Read the model definition and answer for the solid it produces. Units are mm, in the model's axes. A direction names the side the tool comes from. Coordinates: 2 decimals unless noted, no trailing zeros. Write each loop counter-clockwise with the first axis right and the second up, starting at its lowest first coordinate (ties: lowest second). Pieces come first, ordered by that corner, then holes.
1) The part is cut by section D-D (y = -12.25). Determine the outline of the cut face in (x, z).
2) Which of the six approach directions +Z, -Z, +X, -X, +Y, -Y give full straight-line access (tool end or side, diameter ignored) to faces 5 (the face through (7.5, -8, 12)), 6 (the face through (5.5, -6, 12)), 7 (the face through (0, -14.5, 10))?
3) Find the intervals of material crossed by line 1 (X direction, y = -4.5, z = 17); line 2 (Z direction, x = 0, y = -13.4); line 3 (X direction, y = 5.5, z = 11.25), in increasing order.
4) Determine the mould class of faces 1 (the face through (-10.215, 12.199, 12.325)), 2 (the face through (-10, 0, 12)), 3 (the face through (-11.9, 13.93, 12.32)), 4 (the face through (10.199, 12.215, 12.325)) for opening direction X: +X half, -X half, draft (parallel to the pull), parting line (faces both ways), or undercut.
5) Each of these flat-tipped pins is pushed along its axis until it touches: pin 1 Ø6 at (y, z) = (-7, 13.5) entering from +X; pin 2 Ø5.5 at (x, z) = (-1, 12.5) entering from +Y; pin 3 Ø2.5 at (y, z) = (-8.5, 14) entering from -X. Where does it stop, or does it pass through?
6) The part is cut by section C-C (y = 6.5). Determine the outline of the cut face in (x, z), then the cut area to 3 significant figures.
7) The part is cut by section B-B (x = 0). Determine the outline of the cut face in (y, z), then the cut area to 3 significant figures.
from build123d import *

# Parameters (mm, degrees)
F1_DEPTH    = 25
F2_R        = 1.85
F3_DEPTH    = 16.3
F4_T1_DEPTH = 25
F7_R        = 4
F5_DEPTH    = 8.1194955856
F6_DEPTH    = 1.5


# Not quite as in the source:
# - a fillet or chamfer that OpenCascade refuses, or shapes differently, is made with other operations: its cross-section is extruded or revolved along the edge and cut away or added


with BuildPart() as f1:
    # F0 (on Top) → F1 (new body)
    with BuildSketch(Plane.XY):
        with BuildLine():
            Line((-7.5, -2), (-7.5, -14.5))
            Line((-7.5, -14.5), (7.5, -14.5))
            Line((7.5, -14.5), (7.5, -2))
            ThreePointArc((7.5, -2), (8.0857864376, -0.5857864376), (9.5, 0))
            Line((9.5, 0), (10.5, 0))
            ThreePointArc((10.5, 0), (11.9142135624, 0.5857864376), (12.5, 2))
            Line((12.5, 2), (12.5, 12.5))
            ThreePointArc((12.5, 12.5), (11.9142135624, 13.9142135624), (10.5, 14.5))
            Line((10.5, 14.5), (-10.5, 14.5))
            ThreePointArc((-10.5, 14.5), (-11.9142135624, 13.9142135624), (-12.5, 12.5))
            Line((-12.5, 12.5), (-12.5, 2))
            ThreePointArc((-12.5, 2), (-11.9142135624, 0.5857864376), (-10.5, 0))
            Line((-10.5, 0), (-9.5, 0))
            ThreePointArc((-9.5, 0), (-8.0857864376, -0.5857864376), (-7.5, -2))
        make_face()
        with BuildLine():
            Line((-10.5, 1.8729833462), (-10.5, 12.5))
            Line((-10.5, 12.5), (10.5, 12.5))
            Line((10.5, 12.5), (10.5, 1.8729833462))
            ThreePointArc((10.5, 1.8729833462), (7.0505102572, 1.1622776602), (5.5, -2))
            Line((5.5, -2), (5.5, -12.5))
            Line((5.5, -12.5), (-5.5, -12.5))
            Line((-5.5, -12.5), (-5.5, -2))
            ThreePointArc((-5.5, -2), (-7.0505102572, 1.1622776602), (-10.5, 1.8729833462))
        make_face(mode=Mode.SUBTRACT)
    extrude(amount=F1_DEPTH)

    # F2 (on face) → F3 (cut)
    with BuildSketch(Plane.XZ.offset(14.5)):
        with Locations((0, 12.5)):
            Circle(F2_R)
    extrude(amount=-F3_DEPTH, mode=Mode.SUBTRACT)

    # F4: fillet of radius 1 on 4 edges, made by hand

    # F4_s2 → F4_t1 (join)
    with BuildSketch(Plane.XY):
        with BuildLine():
            ThreePointArc((-10.5, 11.5), (-10.2071067812, 12.2071067812), (-9.5, 12.5))
            Line((-9.5, 12.5), (-10.5, 12.5))
            Line((-10.5, 12.5), (-10.5, 11.5))
        make_face()
        with BuildLine():
            ThreePointArc((9.5, 12.5), (10.2071067812, 12.2071067812), (10.5, 11.5))
            Line((10.5, 11.5), (10.5, 12.5))
            Line((10.5, 12.5), (9.5, 12.5))
        make_face()
        with BuildLine():
            ThreePointArc((9.5, 2), (10.2071067812, 2.2928932188), (10.5, 3))
            Line((10.5, 3), (10.5, 1.8729833462))
            ThreePointArc((10.5, 1.8729833462), (10.0040171699, 1.9681187851), (9.5, 2))
        make_face()
        with BuildLine():
            ThreePointArc((-9.5, 2), (-10.2071067812, 2.2928932188), (-10.5, 3))
            Line((-10.5, 3), (-10.5, 1.8729833462))
            ThreePointArc((-10.5, 1.8729833462), (-10.0040171699, 1.9681187851), (-9.5, 2))
        make_face()
    extrude(amount=F4_T1_DEPTH)

    # F7 (on face) → F5 (cut)
    with BuildSketch(Plane(origin=(0, 14.5, 0), x_dir=(-1, 0, 0), z_dir=(0, 1, 0))):
        with Locations((0, 12.5)):
            Circle(F7_R)
    extrude(amount=-F5_DEPTH, mode=Mode.SUBTRACT)

    # F6 (add): a face of the model
    f6_faces = [f1.faces().sort_by_distance(p)[0] for p in [
        (5.2268699943, -12.5, 12.5),
    ]]
    extrude(f6_faces, amount=F6_DEPTH)


solid = f1.part
Reported:
1. outline: (-7.5, 0) - (7.5, 0) - (7.5, 25) - (-7.5, 25) - close; hole circle Ø3.7 at (0, 12.5)
2. face 5: +Z, -Z, +X, -Y
2. face 6: +Z, -Z
2. face 7: +Z, -Z, +X, -X, -Y
3. line 1: x = -7.5 to -5.5, 5.5 to 7.5
3. line 2: z = 0 to 10.65, 14.35 to 25
3. line 3: x = -12.5 to -10.5, 10.5 to 12.5
4. face 1: undercut
4. face 2: draft
4. face 3: -X half
4. face 4: undercut
5. pin 1: stops at x = 7.5
5. pin 2: stops at y = -11
5. pin 3: stops at x = -7.5
6. outline: (-12.5, 0) - (-10.5, 0) - (-10.5, 25) - (-12.5, 25) - close; (10.5, 0) - (12.5, 0) - (12.5, 25) - (10.5, 25) - close
6. area: 100 mm2
7. outline: (-14.5, 0) - (-11, 0) - (-11, 10.65) - (-14.5, 10.65) - close; (-14.5, 14.35) - (-11, 14.35) - (-11, 25) - (-14.5, 25) - close; (12.5, 0) - (14.5, 0) - (14.5, 8.5) - (12.5, 8.5) - close; (12.5, 16.5) - (14.5, 16.5) - (14.5, 25) - (12.5, 25) - close
7. area: 109 mm2
